Geometry check sheet. Reference: drawing and pictorial views, mm from the part's lowest x, y, z. Coordinates: 2 decimals unless noted, no trailing zeros. Loops run counter-clockwise (first coordinate to the right, second up) from the corner with the lowest first, then second, coordinate; pieces in that order, holes last. Notation, with made-up numbers: (60, -36.75) - (65, -36.75) arc R7 cw to (65, -25.75) - close; hole circle Ø1 at (65, 12). An arc over 180 degrees is marked (long way). Use a Markdown table: item, result. Add a question column.
1) Thickness scan on line 1 (Z direction, x = 96, y = 1); line 2 (X direction, y = 1.2, z = 4); line 3 (X direction, y = 0.65, z = 35). Record the ranges inside material, lowest first.
2) Sectioned sample at A-A, the plane z = 25.5. Enter the section's corners in (x, y).
3) Sectioned sample at B-B, the plane y = 0.85. Enter the section's corners in (x, z).
4) Sectioned sample at C-C, the plane x = 28.5. Enter the section's corners in (y, z).
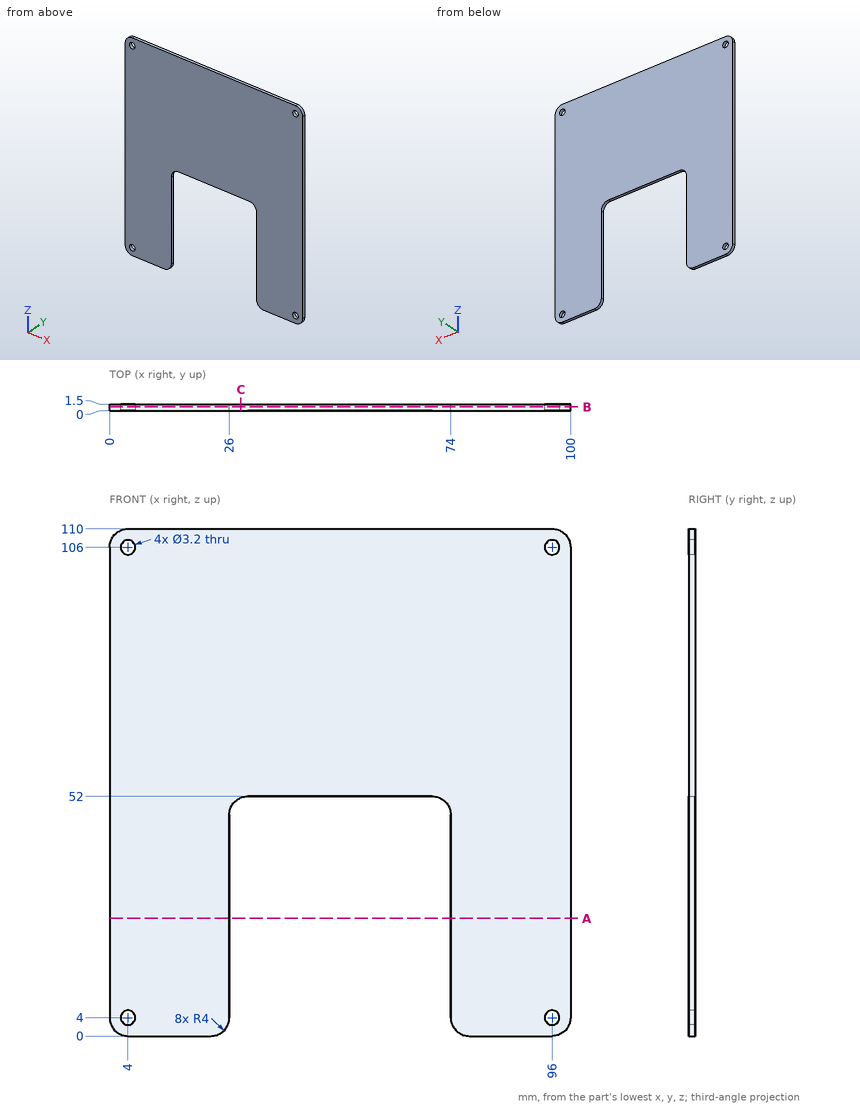
Solved:
| question | item | result |
|---|---|---|
| 1 | line 1 | z = 0 to 2.4, 5.6 to 104.4, 107.6 to 110 |
| 1 | line 2 | x = 0 to 2.4, 5.6 to 26, 74 to 94.4, 97.6 to 100 |
| 1 | line 3 | x = 0 to 26, 74 to 100 |
| 2 | outline | (0, 0) - (26, 0) - (26, 1.5) - (0, 1.5) - close; (74, 0) - (100, 0) - (100, 1.5) - (74, 1.5) - close |
| 3 | outline | (0, 4) arc R4 ccw to (4, 0) - (22, 0) arc R4 ccw to (26, 4) - (26, 48) arc R4 cw to (30, 52) - (70, 52) arc R4 cw to (74, 48) - (74, 4) arc R4 ccw to (78, 0) - (96, 0) arc R4 ccw to (100, 4) - (100, 106) arc R4 ccw to (96, 110) - (4, 110) arc R4 ccw to (0, 106) - close; hole circle Ø3.2 at (4, 4); hole circle Ø3.2 at (4, 106); hole circle Ø3.2 at (96, 4); hole circle Ø3.2 at (96, 106) |
| 4 | outline | (0, 51.71) - (1.5, 51.71) - (1.5, 110) - (0, 110) - close |
